from build123d import *

# Parameters (mm, degrees)
SZKIC1_W = 6
SZKIC1_H = 23.5
SZKIC2_W = 40
SZKIC2_H = 21
SZKIC4_W = 1.8
SZKIC4_H = 2.1
SZKIC5_W = 9
SZKIC5_H = 21
SZKIC8_W = 2.1
SZKIC8_H = 2.1


with BuildPart() as part:
    # Szkic1 → Obr_t1 (revolve)
    with BuildSketch(Plane(origin=(0, 0, 0), x_dir=(0, 0, -1), z_dir=(1, 0, 0)), mode=Mode.PRIVATE) as obr_t1_sk:
        with Locations((-12, 11.75)):
            Rectangle(SZKIC1_W, SZKIC1_H)
    revolve(obr_t1_sk.sketch.rotate(Axis((0, 0, 9), (0, 0, 1)), 270), axis=Axis((0, 0, 9), (0, 0, 1)))

    # Szkic2 → Obr_t2 (revolve)
    with BuildSketch(Plane(origin=(0, 0, 0), x_dir=(0, 0, -1), z_dir=(1, 0, 0)), mode=Mode.PRIVATE) as obr_t2_sk:
        with Locations((-35, 10.5)):
            Rectangle(SZKIC2_W, SZKIC2_H)
    revolve(obr_t2_sk.sketch.rotate(Axis((0, 0, 15), (0, 0, 1)), 270), axis=Axis((0, 0, 15), (0, 0, 1)))

    # Szkic3 → Wyci_cie-obr_t1 (revolve, cut)
    with BuildSketch(Plane(origin=(0, 0, 0), x_dir=(0, 0, -1), z_dir=(1, 0, 0)), mode=Mode.PRIVATE) as wyci_cie_obr_t1_sk:
        Polygon((-55, 20.292893219), (-54.292893219, 21), (-55, 21), align=None)
    revolve(wyci_cie_obr_t1_sk.sketch.rotate(Axis((0, 0, 15), (0, 0, 1)), 270), axis=Axis((0, 0, 15), (0, 0, 1)), mode=Mode.SUBTRACT)

    # Szkic4 → Wyci_cie-obr_t2 (revolve, cut)
    with BuildSketch(Plane(origin=(0, 0, 0), x_dir=(0, 0, -1), z_dir=(1, 0, 0)), mode=Mode.PRIVATE) as wyci_cie_obr_t2_sk:
        with Locations((-15.9, 19.95)):
            Rectangle(SZKIC4_W, SZKIC4_H)
    revolve(wyci_cie_obr_t2_sk.sketch.rotate(Axis((0, 0, 15), (0, 0, 1)), 270), axis=Axis((0, 0, 15), (0, 0, 1)), mode=Mode.SUBTRACT)

    # Szkic5 → Obr_t3 (revolve)
    with BuildSketch(Plane(origin=(0, 0, 0), x_dir=(0, 0, -1), z_dir=(1, 0, 0)), mode=Mode.PRIVATE) as obr_t3_sk:
        with Locations((-4.5, 10.5)):
            Rectangle(SZKIC5_W, SZKIC5_H)
    revolve(obr_t3_sk.sketch.rotate(Axis((0, 0, 0), (0, 0, 1)), 270), axis=Axis((0, 0, 0), (0, 0, 1)))

    # Szkic6 → Wyci_cie-obr_t3 (revolve, cut)
    with BuildSketch(Plane(origin=(0, 0, 0), x_dir=(0, 0, -1), z_dir=(1, 0, 0)), mode=Mode.PRIVATE) as wyci_cie_obr_t3_sk:
        Polygon((-55, 0), (-55, 16), (-1, 16), (0, 17), (0, 0), align=None)
    revolve(wyci_cie_obr_t3_sk.sketch.rotate(Axis((0, 0, 0), (0, 0, 1)), 270), axis=Axis((0, 0, 0), (0, 0, 1)), mode=Mode.SUBTRACT)

    # Szkic7 → Wyci_cie-obr_t4 (revolve, cut)
    with BuildSketch(Plane(origin=(0, 0, 0), x_dir=(0, 0, -1), z_dir=(1, 0, 0)), mode=Mode.PRIVATE) as wyci_cie_obr_t4_sk:
        Polygon((-0.5, 21), (0, 20.5), (0, 21), align=None)
    revolve(wyci_cie_obr_t4_sk.sketch.rotate(Axis((0, 0, 0), (0, 0, 1)), 270), axis=Axis((0, 0, 0), (0, 0, 1)), mode=Mode.SUBTRACT)

    # Szkic8 → Wyci_cie-obr_t5 (revolve, cut)
    with BuildSketch(Plane(origin=(0, 0, 0), x_dir=(0, 0, -1), z_dir=(1, 0, 0)), mode=Mode.PRIVATE) as wyci_cie_obr_t5_sk:
        with Locations((-7.95, 19.95)):
            Rectangle(SZKIC8_W, SZKIC8_H)
    revolve(wyci_cie_obr_t5_sk.sketch.rotate(Axis((0, 0, 0), (0, 0, 1)), 270), axis=Axis((0, 0, 0), (0, 0, 1)), mode=Mode.SUBTRACT)


solid = part.part
For this review, take the finished solid that the model builds, in its own axes (mm). A direction names the side the tool comes from. Round coordinates to 2 decimals unless told otherwise and drop trailing zeros. Loops run counter-clockwise (first coordinate to the right, second up) from the corner with the lowest first, then second, coordinate; pieces in that order, holes last. Notation, with made-up numbers: (48, 60) - (105, 60) arc R23 ccw to (105, 83) - close; hole circle Ø3 at (-13.75, -10.5). An arc over 180 degrees is marked (long way). One line per item, written item: value. Start each with the question number.
Item 1: Take a section at D-D (z = 6). Give the boundary of the cut face in (x, y), plus the area to 3 significant figures.
Item 2: The part is to be moulded in two halves that separate along X. For faces 5 (the cylindrical face through (18.027, 5.677, 15.887)), 6 (the cylindrical face through (-3.47, -15.62, 27.62)), 7 (the flat face through (-3, 17, 0)), say which applies: +X half, -X half, draft (parallel to the pull), parting line (faces both ways), or undercut.
Item 3: For faces 1 (the cylindrical face through (-17.32, 15.88, 11.96)), 2 (the cylindrical face through (20.03, 6.31, 3.66)), 3 (the cylindrical face through (18.027, 5.677, 7.935)), 4 (the cylindrical face through (20.03, 6.31, 35.28)), list the 3-axis set-ups (+Z, -Z, +X, -X, +Y, -Y) from which the entire face can be reached by the end or side of a thin tool; tool diameter is ignored.
Item 4: Take a section at C-C (z = 13.5). Give the boundary of the cut face in (x, y).
Item 5: Clearance check with flat-ended pins moving along their axes: pin 1 Ø5 at (x, z) = (-6.5, 43.5) entering from +Y; pin 2 Ø8 at (x, y) = (14.5, 6.5) entering from -Z; pin 3 Ø4 at (y, z) = (9.5, 14.5) entering from +X; pin 4 Ø12 at (y, z) = (-15, 38) entering from +X. State where each tip first meets the part, or that it passes through.
Item 6: For L1, parallel to Y at x = 0, z = 36; L2, parallel to Z at x = -10.5, y = -18; L3, parallel to X at y = 0.5, z = 50.5, list the stretches that pass through material, from the lowest coordinate up.
Answer below:
1. outline: circle Ø42 at (0, 0); hole circle Ø32 at (0, 0)
1. area: 581 mm2
2. face 5: parting line
2. face 6: undercut
2. face 7: draft
3. face 1: +Z, -Z
3. face 2: -Z
3. face 3: none
3. face 4: +Z
4. outline: circle Ø47 at (0, 0); hole circle Ø32 at (0, 0)
5. pin 1: stops at y = 20.62
5. pin 2: stops at z = 0
5. pin 3: stops at x = 22.27
5. pin 4: stops at x = 18.97
6. L1: y = -21 to -16, 16 to 21
6. L2: z = 0.34 to 6.9, 9 to 15, 16.8 to 54.45
6. L3: x = -20.99 to -15.99, 15.99 to 20.99
